```python
from build123d import *

# Parameters (mm, degrees)
SKETCH_1_W          = 55
SKETCH_1_H          = 10
EXTRUDE_1_DEPTH     = 4
SKETCH_2_W          = 40
SKETCH_2_H          = 10
EXTRUDE_2_DEPTH     = 4
EXTRUDE_3_DEPTH     = 10
EXTRUDE_5_DEPTH     = 10
SKETCH_4_R          = 1.6
CUT_EXTRUDE_1_DEPTH = 5
SKETCH_7_R          = 1.6
CUT_EXTRUDE_2_DEPTH = 4


with BuildPart() as part:
    # ｽｹｯﾁ1 → ﾎﾞｽ - 押し出し1 (new body)
    with BuildSketch(Plane.XY):
        with Locations((4.479686187, -2.540603248)):
            Rectangle(SKETCH_1_W, SKETCH_1_H)
    extrude(amount=EXTRUDE_1_DEPTH)

    # ｽｹｯﾁ2 → ﾎﾞｽ - 押し出し2 (add)
    with BuildSketch(Plane.ZY.offset(23.020313813)):
        with Locations((0, -2.540603248)):
            Rectangle(SKETCH_2_W, SKETCH_2_H)
    extrude(amount=EXTRUDE_2_DEPTH)

    # ｽｹｯﾁ3 → ﾎﾞｽ - 押し出し3 (add)
    with BuildSketch(Plane(origin=(0, 2.459396752, 0), x_dir=(1, 0, 0), z_dir=(0, 1, 0))):
        Polygon((-23.020313813, 5), (-18.020313813, 0), (-23.020313813, 0), align=None)
    extrude(amount=-EXTRUDE_3_DEPTH)

    # ｽｹｯﾁ6 → ﾎﾞｽ - 押し出し5 (add)
    with BuildSketch(Plane.XZ.offset(7.540603248)):
        Polygon((-23.020313813, 9), (-18.020313813, 4), (31.979686187, 4), (31.979686187, 0), (-18.020313813, 0), (-23.020313813, -5), (-23.020313813, -20), (-27.020313813, -20), (-27.020313813, 20), (-23.020313813, 20), align=None)
    extrude(amount=-EXTRUDE_5_DEPTH)

    # ｽｹｯﾁ4 → ｶｯﾄ - 押し出し1 (cut)
    with BuildSketch(Plane.XY.offset(4)):
        with Locations((26.979686187, -2.540603248)):
            Circle(SKETCH_4_R)
        with Locations((21.979686187, -2.540603248)):
            Circle(SKETCH_4_R)
    extrude(amount=-CUT_EXTRUDE_1_DEPTH, mode=Mode.SUBTRACT)

    # ｽｹｯﾁ7 → ｶｯﾄ - 押し出し2 (cut)
    with BuildSketch(Plane(origin=(-23.020313813, 0, 0), x_dir=(0, 0, -1), z_dir=(1, 0, 0))):
        with Locations((-15, -2.540603248)):
            Circle(SKETCH_7_R)
        with Locations((10, -2.540603248)):
            Circle(SKETCH_7_R)
        with Locations((15, -2.540603248)):
            Circle(SKETCH_7_R)
    extrude(amount=-CUT_EXTRUDE_2_DEPTH, mode=Mode.SUBTRACT)


solid = part.part
```
Geometry: final body of the model. Coordinates: model frame, mm. A direction names the side the tool comes from. Coordinates: 2 decimals unless noted, no trailing zeros. Order: outer loops, then holes, each group sorted by start corner. A loop starts at its lowest first (then second) coordinate and runs counter-clockwise, first axis right, second up. Notation, with made-up numbers: (11, 20) - (29, 20) arc R18 ccw to (29, 31) - close; hole circle Ø3 at (-10.5, 36.5). An arc over 180 degrees is marked (long way). Write each question's results on one line, items separated by ' | '.
1) Set-up query: faces 5 (the flat face through (7, -2, 0)), 6 (the cylindrical face through (-25, -2.5, 16.6)), 7 (the flat face through (7, -2, 4)). Return all of +Z, -Z, +X, -X, +Y, -Y with unobstructed straight access to the full face (end or side cutting, diameter ignored); none if empty.
Results list:
face 5: -Z, +X, +Y, -Y | face 6: +X, -X | face 7: +Z, +X, +Y, -Y
2) Pull-direction query (Y, two-part tool) for faces 1 (the cylindrical face through (25.38, -2.47, 2.03)), 2 (the flat face through (-25, -3, 20)), 3 (the flat face through (-8, -7.541, 2)), 4 (the cylindrical face through (-25, -2.5, -13.4)); classes: pulls with the +Y half, pulls with the -Y half, needs draft (parallel to the pull), parting line crosses it, or undercut.
Results list:
face 1: undercut | face 2: needs draft | face 3: pulls with the -Y half | face 4: undercut
3) Section A-A, the plane z = -10. Return loops of the section in (x, y), plus the area to 3 significant figures.
Results list:
outline: (-27.02, -7.54) - (-23.02, -7.54) - (-23.02, -4.14) - (-27.02, -4.14) - close; (-27.02, -0.94) - (-23.02, -0.94) - (-23.02, 2.46) - (-27.02, 2.46) - close | area: 27.2 mm^2
4) Section D-D, the plane z = 1.5. Return loops of the section in (x, y), plus the area to 3 significant figures.
Results list:
outline: (-27.02, -7.54) - (31.98, -7.54) - (31.98, 2.46) - (-27.02, 2.46) - close; hole circle Ø3.2 at (21.98, -2.54); hole circle Ø3.2 at (26.98, -2.54) | area: 574 mm^2
5) Line query: line 1 (Y direction, x = -25.2, z = 15); line 2 (Z direction, x = -10.5, y = 1.25); line 3 (X direction, y = -1.25, z = 1). Output: solid intervals per line, ascending. Write a range as from..to.
Results list:
line 1: -7.54..-4.14, -0.94..2.46 | line 2: 0..4 | line 3: -27.02..21.03, 22.93..26.03, 27.93..31.98
6) Section C-C, the plane y = -3.5. State how many separate pieces and enclosed holes the cut face has, plus the area to 3 significant figures.
Results list:
separate pieces: 6 | enclosed holes: 0 | area: 354 mm^2
7) Pin query (flat end, axial travel): pin 1 (2.5 mm diameter, centred on y = -2.54, z = -15, fed in from +X); pin 2 (5 mm diameter, centred on y = -1, z = -10.5, fed in from +X); pin 3 (6 mm diameter, centred on y = -1.5, z = 15.5, fed in from -X); pin 4 (4 mm diameter, centred on x = 21.98, y = -2.54, fed in from -Z). Return the tip coordinate at first contact, or that it passes through.
Results list:
pin 1: through | pin 2: x = -23.02 | pin 3: x = -27.02 | pin 4: z = 0
8) Section B-B, the plane y = 1. Return loops of the section in (x, z).
Results list:
outline: (-27.02, -20) - (-23.02, -20) - (-23.02, -5) - (-18.02, 0) - (31.98, 0) - (31.98, 4) - (-18.02, 4) - (-23.02, 9) - (-23.02, 20) - (-27.02, 20) - close
